Could you check a few things on this model? Use its own coordinates, in mm. A direction names the side the tool comes from. Give positions to 0.01 mm unless a question says otherwise; leave off trailing zeros. Loops run counter-clockwise (first coordinate to the right, second up) from the corner with the lowest first, then second, coordinate; pieces in that order, holes last. Notation, with made-up numbers: (-38, 56) - (-14, 56) arc R24 ccw to (-14, 84) - close; hole circle Ø1 at (-17.5, -4.75). An arc over 180 degrees is marked (long way). Answer in a Markdown table with one row per item. Add a question column.
```python
from build123d import *

# Parameters (mm, degrees)
SKETCH1_W          = 6
SKETCH1_H          = 2
CUT_EXTRUDE1_DEPTH = 2.3
CHAMFER1_SIZE      = 0.75
CHAMFER2_SIZE      = 0.2


with BuildPart() as part:
    # Sketch1 → Revolve1 (revolve)
    with BuildSketch(Plane(origin=(0, 0, 0), x_dir=(-1, 0, 0), z_dir=(0, 0, -1)), mode=Mode.PRIVATE) as revolve1_sk:
        with Locations((-3, 1)):
            Rectangle(SKETCH1_W, SKETCH1_H)
    revolve(revolve1_sk.sketch.rotate(Axis((6, 0, 0), (-1, 0, 0)), 270), axis=Axis((6, 0, 0), (-1, 0, 0)))

    # Sketch2 → Cut-Extrude1 (cut)
    with BuildSketch(Plane.ZY):
        Polygon((0.577350269, -1), (1.154700538, 0), (0.577350269, 1), (-0.577350269, 1), (-1.154700538, 0), (-0.577350269, -1), align=None)
    extrude(amount=-CUT_EXTRUDE1_DEPTH, mode=Mode.SUBTRACT)

    # Chamfer1
    chamfer1_edges = [part.edges().sort_by_distance(p)[0] for p in [
        (6, 0, -2),
    ]]
    chamfer(chamfer1_edges, length=CHAMFER1_SIZE)

    # Chamfer2
    chamfer2_edges = [part.edges().sort_by_distance(p)[0] for p in [
        (0, 0, -2),
    ]]
    chamfer(chamfer2_edges, length=CHAMFER2_SIZE)


solid = part.part
```
(1) I want a section at C-C on x = 2.95. Please give me the cut outline in (y, z), then the cut area to 3 significant figures.
(2) I want a section at B-B on z = 0. Please give me the cut outline in (x, y), then the cut area to 3 significant figures.
(3) On a 3-axis mill with a long thin cutter (end or side, diameter ignored), from which of +Z, -Z, +X, -X, +Y, -Y can I reach the whole of each face in a straight line? I mean faces 5 (the flat face through (0, -1, -1)), 6 (the flat face through (1.13, 0.51, -0.86)). Say none if no direction works.
(4) I want a section at A-A on x = 2.05. Please give me the cut outline in (y, z).
(5) We'd pull the mould along Z, two halves only. Please class faces 1 (the cylindrical face through (3, -2, 0)), 2 (the flat face through (6, 0, 0)), 3 (the flat face through (1.13, 0.49, 0.87)), 4 (the flat face through (1.13, -0.49, -0.87)): pulls with the +Z half, pulls with the -Z half, needs draft (parallel to the pull), parting line crosses it, or undercut.
(6) Please list where these lines run through material, in increasing order: line 1 (X direction, y = 0, z = 1); line 2 (Z direction, x = 1.5, y = 0.8); line 3 (Y direction, x = 0.4, z = -1.1).
Reported:
| question | item | result |
|---|---|---|
| 1 | outline | circle Ø4 at (0, 0) |
| 1 | area | 12.6 mm² |
| 2 | outline | (0, -1.8) - (0.2, -2) - (5.25, -2) - (6, -1.25) - (6, 1.25) - (5.25, 2) - (0.2, 2) - (0, 1.8) - (0, 1) - (2.3, 1) - (2.3, -1) - (0, -1) - close |
| 2 | area | 18.8 mm² |
| 3 | face 5 | +Z, -Z, -X, +Y, -Y |
| 3 | face 6 | -X |
| 4 | outline | circle Ø4 at (0, 0); hole (-1, -0.58) - (0, -1.15) - (1, -0.58) - (1, 0.58) - (0, 1.15) - (-1, 0.58) - close |
| 5 | face 1 | parting line crosses it |
| 5 | face 2 | needs draft |
| 5 | face 3 | undercut |
| 5 | face 4 | undercut |
| 6 | line 1 | 2.3 to 6 |
| 6 | line 2 | -1.83 to -0.69, 0.69 to 1.83 |
| 6 | line 3 | -1.67 to -0.09, 0.09 to 1.67 |
